```python
from build123d import *

# Parameters (mm, degrees)
BOSS_EXTRUDE2_DEPTH     = 26.9875
SKETCH3_W               = 62.061672923
SKETCH3_H               = 40.225982375
CUT_EXTRUDE1_DEPTH      = 39.1
CUT_EXTRUDE1_DEPTH_BACK = 51.8
SKETCH4_W               = 6.35
SKETCH4_H               = 40.225982375
CUT_EXTRUDE2_DEPTH      = 31.75
BOSS_EXTRUDE3_DEPTH     = 4.7625


with BuildPart() as part:
    # Sketch1 → Boss-Extrude2 (new body, symmetric)
    with BuildSketch(Plane.XY):
        with BuildLine():
            Line((66.675, 0), (-6.35, 0))
            ThreePointArc((-6.35, 0), (-9.986642245, 0.531810604), (-13.318716788, 2.082703436))
            Line((-13.318716788, 2.082703436), (-66.971034996, 37.297676322))
            ThreePointArc((-66.971034996, 37.297676322), (-68.46461012, 37.896146949), (-70.06066077, 38.1))
            Line((-70.06066077, 38.1), (-74.761672923, 38.1))
            ThreePointArc((-74.761672923, 38.1), (-79.251800983, 36.240128061), (-81.111672923, 31.75))
            Line((-81.111672923, 31.75), (-81.111672923, 21.961704715))
            ThreePointArc((-81.111672923, 21.961704715), (-80.533790997, 19.314979768), (-78.90532554, 17.149985376))
            Line((-78.90532554, 17.149985376), (0, -50.8))
            Line((0, -50.8), (0, -6.35))
            Line((0, -6.35), (60.325, -6.35))
            ThreePointArc((60.325, -6.35), (64.815128061, -4.490128061), (66.675, 0))
        make_face()
    extrude(amount=BOSS_EXTRUDE2_DEPTH, both=True)

    # Sketch3 → Cut-Extrude1 (cut, two sides)
    with BuildSketch(Plane(origin=(0, 0, 0), x_dir=(1, 0, 0), z_dir=(0, 1, 0))) as cut_extrude1_sk:
        with Locations((-37.380836461, -0.195905759)):
            Rectangle(SKETCH3_W, SKETCH3_H)
    extrude(amount=CUT_EXTRUDE1_DEPTH, mode=Mode.SUBTRACT)
    extrude(cut_extrude1_sk.sketch, amount=-CUT_EXTRUDE1_DEPTH_BACK, mode=Mode.SUBTRACT)

    # Sketch4 → Cut-Extrude2 (cut)
    with BuildSketch(Plane(origin=(0, 0, 0), x_dir=(1, 0, 0), z_dir=(0, 1, 0))):
        with Locations((-71.586672923, -0.195905759)):
            Rectangle(SKETCH4_W, SKETCH4_H)
    extrude(amount=CUT_EXTRUDE2_DEPTH, mode=Mode.SUBTRACT)

    # Sketch5 → Boss-Extrude3 (add, symmetric)
    with BuildSketch(Plane.XY):
        Polygon((0, -50.8), (44.45, -6.35), (0, -6.35), align=None)
    extrude(amount=BOSS_EXTRUDE3_DEPTH, both=True)


solid = part.part
```
Work out the finished part from the listing and answer in its coordinate system (mm). A direction names the side the tool comes from. Round coordinates to 2 decimals unless told otherwise and drop trailing zeros. Write each loop counter-clockwise with the first axis right and the second up, starting at its lowest first coordinate (ties: lowest second). Pieces come first, ordered by that corner, then holes.
1) A cutting plane is placed at D-D on z = -22. Determine the outline of the cut face in (x, y) (3 decimals), and give its area (3 significant figures).
2) Flat-ended cylindrical pins translate along their axes: P1, Ø20, axis at y = 26.5, z = -6, coming from the +X side; P2, Ø6, axis at y = -39.5, z = 14.5, coming from the +X side; P3, Ø13.5, axis at x = 30, y = -29, coming from the -Z side. Find the tip coordinate at first contact, or state that the pin passes through.
3) Which of the six approach directions +Z, -Z, +X, -X, +Y, -Y give full straight-line access (tool end or side, diameter ignored) to faces 1 (the face through (-80.55, 19.35, 0.38)), 2 (the face through (-6.35, -22, 0)), 3 (the face through (0, -29, 16)), 4 (the face through (31, 0, 0)), 5 (the face through (30, -6.35, 6))?
4) Determine the mould class of faces 6 (the face through (-29, 0, -26.988)), 7 (the face through (-68.412, 35, 0)), 8 (the face through (-41, -4, 20.309)), 9 (the face through (21.9, -28.9, 0.1)) for opening direction Z: pulls with the +Z half, pulls with the -Z half, needs draft (parallel to the pull), parting line crosses it, or undercut.
5) A cutting plane is placed at C-C on y = 10.5. Determine the outline of the cut face in (x, z), and give its area (3 significant figures).
6) A cutting plane is placed at B-B on x = 11. Determine the outline of the cut face in (y, z), and give its area (3 significant figures).
7) A cutting plane is placed at A-A on z = -3. Determine the outline of the cut face in (x, y) (3 decimals), and give its area (3 significant figures).
8) Consider probe 1 along Z at (x, y) = (-14, -1); probe 2 along X at (y, z) = (-29, 16). Determine where each line is inside the solid, lowest interval first.
Entries:
1. outline: (-81.112, 21.962) arc R6.35 ccw to (-78.905, 17.15) - (0, -50.8) - (0, -6.35) - (60.325, -6.35) arc R6.35 ccw to (66.675, 0) - (-6.35, 0) arc R12.7 cw to (-13.319, 2.083) - (-66.971, 37.298) arc R6.35 ccw to (-70.061, 38.1) - (-74.762, 38.1) arc R6.35 ccw to (-81.112, 31.75) - close
1. area: 3,290 mm2
2. P1: stops at x = -68.41
2. P2: stops at x = 0
2. P3: stops at z = -4.76
3. face 1: +Z, -Z, -X, -Y
3. face 2: -X, +Y, -Y
3. face 3: +Z, +X, -Y
3. face 4: +Z, -Z, +X, +Y
3. face 5: +X, -Y
4. face 6: pulls with the -Z half
4. face 7: undercut
4. face 8: undercut
4. face 9: needs draft
5. outline: (-71.18, -26.99) - (-26.14, -26.99) - (-26.14, -19.92) - (-71.18, -19.92) - close; (-71.18, 20.31) - (-26.14, 20.31) - (-26.14, 26.99) - (-71.18, 26.99) - close
5. area: 619 mm2
6. outline: (-39.8, -4.76) - (-6.35, -4.76) - (-6.35, -26.99) - (0, -26.99) - (0, 26.99) - (-6.35, 26.99) - (-6.35, 4.76) - (-39.8, 4.76) - close
6. area: 661 mm2
7. outline: (-81.112, 21.962) arc R6.35 ccw to (-78.905, 17.15) - (-74.762, 13.582) - (-74.762, 31.75) - (-68.412, 31.75) - (-68.412, 37.882) arc R6.35 ccw to (-70.061, 38.1) - (-74.762, 38.1) arc R6.35 ccw to (-81.112, 31.75) - close; (-6.35, -45.332) - (0, -50.8) - (44.45, -6.35) - (60.325, -6.35) arc R6.35 ccw to (66.675, 0) - (-6.35, 0) - close
7. area: 1,880 mm2
8. probe 1: z = -26.99 to -19.92, 20.31 to 26.99
8. probe 2: x = -6.35 to 0
